Build history of the part. All positions in model axes, mm. Round coordinates to 2 decimals unless told otherwise and drop trailing zeros. Write each loop counter-clockwise with the first axis right and the second up, starting at its lowest first coordinate (ties: lowest second). Pieces come first, ordered by that corner, then holes. Notation, with made-up numbers: (-5.5, -31) -> (26.5, -31) arc R6 ccw to (26.5, -20) -> close; hole circle Ø6 at (12, 10.5). An arc over 180 degrees is marked (long way). One line per question, with ' | ' between items.
from build123d import *

# Parameters (mm, degrees)
ESQUISSE1_W        = 13
ESQUISSE1_H        = 13
ESQUISSE1_R        = 2.1
BOSS_EXTRU_1_DEPTH = 2
CONG_1_R           = 2
CONG_2_R           = 0.5


with BuildPart() as part:
    # Esquisse1 → Boss.-Extru.1 (new body)
    with BuildSketch(Plane.XY):
        with Locations((-5.035571526, 2.289308176)):
            Rectangle(ESQUISSE1_W, ESQUISSE1_H)
        with Locations((-5.035571526, 2.289308176)):
            Circle(ESQUISSE1_R, mode=Mode.SUBTRACT)
    extrude(amount=BOSS_EXTRU_1_DEPTH)

    # Congé1
    cong_1_edges = [part.edges().sort_by_distance(p)[0] for p in [
        (1.464428474, -4.210691824, 1),
        (-11.535571526, -4.210691824, 1),
        (-11.535571526, 8.789308176, 1),
        (1.464428474, 8.789308176, 1),
    ]]
    fillet(cong_1_edges, radius=CONG_1_R)

    # Congé2
    cong_2_edges = [part.edges().sort_by_distance(p)[0] for p in [
        (-7.135571526, 2.289308176, 2),
        (-5.035571526, -4.210691824, 2),
        (-11.535571526, 2.289308176, 2),
        (1.464428474, 2.289308176, 2),
        (-5.035571526, 8.789308176, 2),
        (0.878642036, 8.203521738, 2),
        (-10.949785089, 8.203521738, 2),
        (0.878642036, -3.624905386, 2),
        (-10.949785089, -3.624905386, 2),
    ]]
    fillet(cong_2_edges, radius=CONG_2_R)


solid = part.part
(1) Drop a flat-ended pin along its axis: pin 1 (2.5 mm diameter, centred on x = -5.04, y = 2.29, fed in from -Z). Give the stop position or say it passes through.
Calculated:
pin 1: through
(2) Slice it at A-A (z = 0.3). Write the cut outline in (x, y).
Calculated:
outline: (-11.54, -2.21) arc R2 ccw to (-9.54, -4.21) -> (-0.54, -4.21) arc R2 ccw to (1.46, -2.21) -> (1.46, 6.79) arc R2 ccw to (-0.54, 8.79) -> (-9.54, 8.79) arc R2 ccw to (-11.54, 6.79) -> close; hole circle Ø4.2 at (-5.04, 2.29)
(3) Mould opens along X. For faces 1 (the flat face through (-5, 8.789, 1)), 2 (the cylindrical face through (-10.965, -3.609, 0.76)), 3 (the cylindrical face through (-6.7, 1.01, 0.74)) say: pulls with the +X half, pulls with the -X half, needs draft (parallel to the pull), parting line crosses it, or undercut.
Calculated:
face 1: needs draft | face 2: pulls with the -X half | face 3: undercut
(4) Wall check: line 1 (Y direction, x = -6.5, z = 1); line 2 (X direction, y = 1.5, z = 0.25); line 3 (X direction, y = 1.75, z = 0.75). Give the ranges that are in metal, low to high. Write a range as from..to.
Calculated:
line 1: -4.21..0.78, 3.79..8.79 | line 2: -11.54..-6.98, -3.09..1.46 | line 3: -11.54..-7.07, -3.01..1.46
